from build123d import *

# Parameters (mm, degrees)
SKETCH_1_W               = 110
SKETCH_1_H               = 10
EXTRUDE_1_DEPTH          = 10
CUT_EXTRUDE_1_DEPTH      = 57.124860802
CUT_EXTRUDE_1_DEPTH_BACK = 57.124860802
SKETCH_2_R               = 1.5


with BuildPart() as part:
    # ｽｹｯﾁ1 → ﾎﾞｽ - 押し出し1 (new body)
    with BuildSketch(Plane(origin=(0, 0, 0), x_dir=(1, 0, 0), z_dir=(0, 1, 0))):
        Rectangle(SKETCH_1_W, SKETCH_1_H)
    extrude(amount=EXTRUDE_1_DEPTH)

    # ｽｹｯﾁ2 → ｶｯﾄ - 押し出し1 (cut, two sides: drawn at the far end of the back side and taken through both)
    with BuildSketch(Plane(origin=(0, 0, 0), x_dir=(0, 0, -1), z_dir=(1, 0, 0)).offset(-CUT_EXTRUDE_1_DEPTH_BACK)):
        with Locations((0, 5)):
            Circle(SKETCH_2_R)
    extrude(amount=CUT_EXTRUDE_1_DEPTH + CUT_EXTRUDE_1_DEPTH_BACK, mode=Mode.SUBTRACT)


solid = part.part
Could you check a few things on this model? Use its own coordinates, in mm. Give positions to 0.01 mm unless a question says otherwise; leave off trailing zeros. Write each loop counter-clockwise with the first axis right and the second up, starting at its lowest first coordinate (ties: lowest second). Pieces come first, ordered by that corner, then holes. Notation, with made-up numbers: (73, 71.5) -> (127, 71.5) arc R24 cw to (127, 90.5) -> close; hole circle Ø10 at (75, 34). An arc over 180 degrees is marked (long way). Answer as CSV lines item,"result". Start each with the question number.
(1) If we section it at A-A, the plane y = 5: Write out the boundary of the cut face in (x, z), and give its area (3 significant figures).
(2) If we section it at B-B, the plane z = 0: Write out the boundary of the cut face in (x, y), and give its area (3 significant figures).
(3) If we section it at C-C, the plane x = -5: Write out the boundary of the cut face in (y, z).
(4) Please list where these lines run through material, in increasing order: line 1 (Z direction, x = 28, y = 5); line 2 (Y direction, x = -39.5, z = 0.25); line 3 (Z direction, x = 17, y = 3.75).
(5) If we mould it in two halves opening along Z, with no side actions, what happens to faces 1 (the face through (-1, 10, 0)), 2 (the face through (-1, 5, -5)), 3 (the face through (-0.77, 5.07, 1.5))? For each: +Z half, -Z half, draft (parallel to the pull), parting line (faces both ways), or undercut.
Answer list:
1,outline,"(-55, -5) -> (55, -5) -> (55, -1.5) -> (-55, -1.5) -> close; (-55, 1.5) -> (55, 1.5) -> (55, 5) -> (-55, 5) -> close"
1,area,"770 mm^2"
2,outline,"(-55, 0) -> (55, 0) -> (55, 3.5) -> (-55, 3.5) -> close; (-55, 6.5) -> (55, 6.5) -> (55, 10) -> (-55, 10) -> close"
2,area,"770 mm^2"
3,outline,"(0, -5) -> (10, -5) -> (10, 5) -> (0, 5) -> close; hole circle Ø3 at (5, 0)"
4,line 1,"-5 to -1.5, 1.5 to 5"
4,line 2,"0 to 3.52, 6.48 to 10"
4,line 3,"-5 to -0.83, 0.83 to 5"
5,face 1,"draft"
5,face 2,"-Z half"
5,face 3,"undercut"
